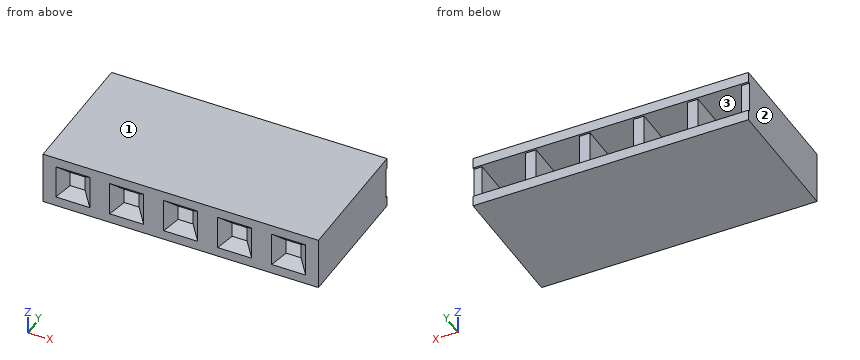
```python
from build123d import *

# Parameters (mm, degrees)
SKETCH1_W                 = 12.96
SKETCH1_H                 = 2.5
BOSS_EXTRUDE1_DEPTH       = 6.2
SKETCH2_W                 = 2.04
SKETCH2_H                 = 1.5
CUT_EXTRUDE1_DEPTH        = 5.75
SKETCH3_W                 = 1.6
SKETCH3_H                 = 1.6
CUT_EXTRUDE2_DEPTH        = 0.45
CUT_EXTRUDE2_DRAFT        = -45
LPATTERN1_COUNT           = 5
LPATTERN1_PITCH           = 2.54
LPATTERN1_COPY_1_SKETCH_W = 1.6
LPATTERN1_COPY_1_SKETCH_H = 1.6
LPATTERN1_COPY_1_DEPTH    = 0.45
LPATTERN1_COPY_1_DRAFT    = -45
LPATTERN1_COPY_2_SKETCH_W = 1.6
LPATTERN1_COPY_2_SKETCH_H = 1.6
LPATTERN1_COPY_2_DEPTH    = 0.45
LPATTERN1_COPY_2_DRAFT    = -45
LPATTERN1_COPY_3_SKETCH_W = 1.6
LPATTERN1_COPY_3_SKETCH_H = 1.6
LPATTERN1_COPY_3_DEPTH    = 0.45
LPATTERN1_COPY_3_DRAFT    = -45
LPATTERN1_COPY_4_SKETCH_W = 1.6
LPATTERN1_COPY_4_SKETCH_H = 1.6
LPATTERN1_COPY_4_DEPTH    = 0.45
LPATTERN1_COPY_4_DRAFT    = -45
SKETCH4_W                 = 12.96
SKETCH4_H                 = 0.5
BOSS_EXTRUDE2_DEPTH       = 0.1


with BuildPart() as part:
    # Sketch1 → Boss-Extrude1 (new body)
    with BuildSketch(Plane(origin=(0, 0, 0), x_dir=(1, 0, 0), z_dir=(0, 1, 0))):
        Rectangle(SKETCH1_W, SKETCH1_H)
    extrude(amount=BOSS_EXTRUDE1_DEPTH)

    # Sketch2 → Cut-Extrude1 (cut)
    with BuildSketch(Plane(origin=(0, 6.2, 0), x_dir=(1, 0, 0), z_dir=(0, 1, 0))):
        with Locations((-5.08, 0)):
            Rectangle(SKETCH2_W, SKETCH2_H)
    cut_extrude1 = extrude(amount=-CUT_EXTRUDE1_DEPTH, mode=Mode.SUBTRACT)


with BuildPart() as cut_extrude2_tool:
    # Sketch3 → Cut-Extrude2 (with draft: the straight prism first)
    with BuildSketch(Plane.XZ):
        with Locations((-5.08, 0)):
            Rectangle(SKETCH3_W, SKETCH3_H)
    extrude(amount=-CUT_EXTRUDE2_DEPTH)
    # Cut-Extrude2: the draft: its side faces are tilted about the plane it starts from
    cut_extrude2_sides = [cut_extrude2_tool.faces().sort_by_distance(p)[0] for p in [
        (-5.08, 0.225, -0.8),
        (-4.28, 0.225, 0),
        (-5.08, 0.225, 0.8),
        (-5.88, 0.225, 0),
    ]]
    draft(cut_extrude2_sides, Plane.XZ, CUT_EXTRUDE2_DRAFT)


with BuildPart() as part_1:
    add(part.part)

    # Cut-Extrude2: cut by cut_extrude2_tool
    add(cut_extrude2_tool.part, mode=Mode.SUBTRACT)

    # LPattern1: Cut-Extrude1 ×5
    with Locations(*[(i * LPATTERN1_PITCH, 0, 0) for i in range(1, LPATTERN1_COUNT)]):
        add(cut_extrude1, mode=Mode.SUBTRACT)


with BuildPart() as lpattern1_copy_1_tool:
    # LPattern1 copy 1 sketch → LPattern1 copy 1 (with draft: the straight prism first)
    with BuildSketch(Plane(origin=(2.54, 0, 0), x_dir=(1, 0, 0), z_dir=(0, -1, 0))):
        with Locations((-5.08, 0)):
            Rectangle(LPATTERN1_COPY_1_SKETCH_W, LPATTERN1_COPY_1_SKETCH_H)
    extrude(amount=-LPATTERN1_COPY_1_DEPTH)
    # LPattern1 copy 1: the draft: its side faces are tilted about the plane it starts from
    lpattern1_copy_1_sides = [lpattern1_copy_1_tool.faces().sort_by_distance(p)[0] for p in [
        (-2.54, 0.225, -0.8),
        (-1.74, 0.225, 0),
        (-2.54, 0.225, 0.8),
        (-3.34, 0.225, 0),
    ]]
    draft(lpattern1_copy_1_sides, Plane(origin=(2.54, 0, 0), x_dir=(1, 0, 0), z_dir=(0, -1, 0)), LPATTERN1_COPY_1_DRAFT)


with BuildPart() as part_2:
    add(part_1.part)

    # LPattern1 copy 1: cut by lpattern1_copy_1_tool
    add(lpattern1_copy_1_tool.part, mode=Mode.SUBTRACT)


with BuildPart() as lpattern1_copy_2_tool:
    # LPattern1 copy 2 sketch → LPattern1 copy 2 (with draft: the straight prism first)
    with BuildSketch(Plane(origin=(5.08, 0, 0), x_dir=(1, 0, 0), z_dir=(0, -1, 0))):
        with Locations((-5.08, 0)):
            Rectangle(LPATTERN1_COPY_2_SKETCH_W, LPATTERN1_COPY_2_SKETCH_H)
    extrude(amount=-LPATTERN1_COPY_2_DEPTH)
    # LPattern1 copy 2: the draft: its side faces are tilted about the plane it starts from
    lpattern1_copy_2_sides = [lpattern1_copy_2_tool.faces().sort_by_distance(p)[0] for p in [
        (0, 0.225, -0.8),
        (0.8, 0.225, 0),
        (0, 0.225, 0.8),
        (-0.8, 0.225, 0),
    ]]
    draft(lpattern1_copy_2_sides, Plane(origin=(5.08, 0, 0), x_dir=(1, 0, 0), z_dir=(0, -1, 0)), LPATTERN1_COPY_2_DRAFT)


with BuildPart() as part_3:
    add(part_2.part)

    # LPattern1 copy 2: cut by lpattern1_copy_2_tool
    add(lpattern1_copy_2_tool.part, mode=Mode.SUBTRACT)


with BuildPart() as lpattern1_copy_3_tool:
    # LPattern1 copy 3 sketch → LPattern1 copy 3 (with draft: the straight prism first)
    with BuildSketch(Plane(origin=(7.62, 0, 0), x_dir=(1, 0, 0), z_dir=(0, -1, 0))):
        with Locations((-5.08, 0)):
            Rectangle(LPATTERN1_COPY_3_SKETCH_W, LPATTERN1_COPY_3_SKETCH_H)
    extrude(amount=-LPATTERN1_COPY_3_DEPTH)
    # LPattern1 copy 3: the draft: its side faces are tilted about the plane it starts from
    lpattern1_copy_3_sides = [lpattern1_copy_3_tool.faces().sort_by_distance(p)[0] for p in [
        (2.54, 0.225, -0.8),
        (3.34, 0.225, 0),
        (2.54, 0.225, 0.8),
        (1.74, 0.225, 0),
    ]]
    draft(lpattern1_copy_3_sides, Plane(origin=(7.62, 0, 0), x_dir=(1, 0, 0), z_dir=(0, -1, 0)), LPATTERN1_COPY_3_DRAFT)


with BuildPart() as part_4:
    add(part_3.part)

    # LPattern1 copy 3: cut by lpattern1_copy_3_tool
    add(lpattern1_copy_3_tool.part, mode=Mode.SUBTRACT)


with BuildPart() as lpattern1_copy_4_tool:
    # LPattern1 copy 4 sketch → LPattern1 copy 4 (with draft: the straight prism first)
    with BuildSketch(Plane(origin=(10.16, 0, 0), x_dir=(1, 0, 0), z_dir=(0, -1, 0))):
        with Locations((-5.08, 0)):
            Rectangle(LPATTERN1_COPY_4_SKETCH_W, LPATTERN1_COPY_4_SKETCH_H)
    extrude(amount=-LPATTERN1_COPY_4_DEPTH)
    # LPattern1 copy 4: the draft: its side faces are tilted about the plane it starts from
    lpattern1_copy_4_sides = [lpattern1_copy_4_tool.faces().sort_by_distance(p)[0] for p in [
        (5.08, 0.225, -0.8),
        (5.88, 0.225, 0),
        (5.08, 0.225, 0.8),
        (4.28, 0.225, 0),
    ]]
    draft(lpattern1_copy_4_sides, Plane(origin=(10.16, 0, 0), x_dir=(1, 0, 0), z_dir=(0, -1, 0)), LPATTERN1_COPY_4_DRAFT)


with BuildPart() as part_5:
    add(part_4.part)

    # LPattern1 copy 4: cut by lpattern1_copy_4_tool
    add(lpattern1_copy_4_tool.part, mode=Mode.SUBTRACT)

    # Sketch4 → Boss-Extrude2 (add)
    with BuildSketch(Plane(origin=(0, 6.2, 0), x_dir=(1, 0, 0), z_dir=(0, 1, 0))):
        with Locations((0, 1)):
            Rectangle(SKETCH4_W, SKETCH4_H)
    boss_extrude2 = extrude(amount=BOSS_EXTRUDE2_DEPTH)

    # Mirror1: Boss-Extrude2 across plane
    add(boss_extrude2.mirror(Plane.XY))


solid = part_5.part
```
Input: part model. Units: mm. Frame: model coordinates. Face numbers are marked on the shaded views. Round coordinates to 2 decimals unless told otherwise and drop trailing zeros. Order: outer loops, then holes, each group sorted by start corner. A loop starts at its lowest first (then second) coordinate and runs counter-clockwise, first axis right, second up. Notation, with made-up numbers: (9.25, 6.25) - (19.25, 6.25) arc R34 cw to (19.25, 36.25) - close; hole circle Ø6 at (-10.5, -21). An arc over 180 degrees is marked (long way). Answer in a Markdown table with one row per item.
Item 1: Section query A-A (x = 0). Return the cut outline in (y, z), then the cut area to 3 significant figures.
Model answer:
| item | result |
|---|---|
| outline | (0, -1.25) - (6.3, -1.25) - (6.3, -0.75) - (0.45, -0.75) - (0.45, -0.35) - (0, -0.8) - close; (0, 0.8) - (0.45, 0.35) - (0.45, 0.75) - (6.3, 0.75) - (6.3, 1.25) - (0, 1.25) - close |
| area | 6.46 mm² |
Item 2: Line query: line 1 (X direction, y = 6, z = 0.35); line 2 (Z direction, x = -2.5, y = 4.5); line 3 (Y direction, x = 1.25, z = 0.35). Output: solid intervals per line, ascending.
Model answer:
| item | result |
|---|---|
| line 1 | x = -6.48 to -6.1, -4.06 to -3.56, -1.52 to -1.02, 1.02 to 1.52, 3.56 to 4.06, 6.1 to 6.48 |
| line 2 | z = -1.25 to -0.75, 0.75 to 1.25 |
| line 3 | y = 0 to 6.2 |
Item 3: Pin query (flat end, axial travel): pin 1 (1.2 mm diameter, centred on x = 3, z = 0, fed in from +Y). Return the tip coordinate at first contact, or that it passes through.
Model answer:
| item | result |
|---|---|
| pin 1 | stops at y = 6.2 |
Item 4: Section query C-C (z = -0.15). Give the number of separate pieces and of enclosed holes in the cut face, then the cut area to 3 significant figures.
Model answer:
| item | result |
|---|---|
| separate pieces | 6 |
| enclosed holes | 0 |
| area | 19.1 mm² |
Item 5: Section query D-D (x = 2). Return the cut outline in (y, z).
Model answer:
| item | result |
|---|---|
| outline | (0, -1.25) - (6.3, -1.25) - (6.3, -0.75) - (0.45, -0.75) - (0.45, 0.75) - (6.3, 0.75) - (6.3, 1.25) - (0, 1.25) - (0, 0.8) - (0.26, 0.54) - (0.26, -0.54) - (0, -0.8) - close |
Item 6: Mould query, pull axis X, two halves, no side actions, for the marked faces 1, 2 and 3. Classes: released by +X, released by -X, zero draft, split by the parting line, or undercut.
Model answer:
| item | result |
|---|---|
| face 1 | zero draft |
| face 2 | released by -X |
| face 3 | undercut |
Item 7: Section query B-B (y = 1). Return the cut outline in (x, z), then the cut area to 3 significant figures.
Model answer:
| item | result |
|---|---|
| outline | (-6.48, -1.25) - (6.48, -1.25) - (6.48, 1.25) - (-6.48, 1.25) - close; hole (-6.1, -0.75) - (-4.06, -0.75) - (-4.06, 0.75) - (-6.1, 0.75) - close; hole (-3.56, -0.75) - (-1.52, -0.75) - (-1.52, 0.75) - (-3.56, 0.75) - close; hole (-1.02, -0.75) - (1.02, -0.75) - (1.02, 0.75) - (-1.02, 0.75) - close; hole (1.52, -0.75) - (3.56, -0.75) - (3.56, 0.75) - (1.52, 0.75) - close; hole (4.06, -0.75) - (6.1, -0.75) - (6.1, 0.75) - (4.06, 0.75) - close |
| area | 17.1 mm² |
